from build123d import *

# Parameters (mm, degrees)
BOSS_EXTRUDE1_DEPTH = 90
SKETCH2_R           = 10
CUT_EXTRUDE1_DEPTH  = 90
CUT_EXTRUDE2_DEPTH  = 10
CUT_EXTRUDE3_DEPTH  = 20
SKETCH11_W          = 10
SKETCH11_H          = 9.986072288
BOSS_EXTRUDE2_DEPTH = 70
SKETCH12_W          = 20
SKETCH12_H          = 9.986072288
CUT_EXTRUDE11_DEPTH = 10
CUT_EXTRUDE25_DEPTH = 30
CUT_EXTRUDE26_DEPTH = 30
CUT_EXTRUDE27_DEPTH = 83


with BuildPart() as part:
    # Sketch1 → Boss-Extrude1 (new body)
    with BuildSketch(Plane(origin=(0, 0, 0), x_dir=(1, 0, 0), z_dir=(0, 1, 0))):
        with BuildLine():
            Line((-40, 0), (-30, 0))
            Line((-30, 0), (-30, -30))
            Line((-30, -30), (0, -30))
            Line((0, -30), (20, -50))
            Line((20, -50), (40, -50))
            Line((40, -50), (40, 0))
            ThreePointArc((40, 0), (0, 40), (-40, 0))
        make_face()
    extrude(amount=BOSS_EXTRUDE1_DEPTH)

    # Sketch2 → Cut-Extrude1 (cut)
    with BuildSketch(Plane(origin=(0, 90, 0), x_dir=(1, 0, 0), z_dir=(0, 1, 0))):
        with Locations(Location((0, 0, 0), (0, 0, 270))):
            Circle(SKETCH2_R)
    extrude(amount=-CUT_EXTRUDE1_DEPTH, mode=Mode.SUBTRACT)

    # Sketch3 → Cut-Extrude2 (cut)
    with BuildSketch(Plane(origin=(0, 90, 0), x_dir=(1, 0, 0), z_dir=(0, 1, 0))):
        with BuildLine():
            Line((30, 0), (40, 0))
            Line((40, 0), (40, -40))
            Line((40, -40), (20, -20))
            Line((20, -20), (20, 0))
            ThreePointArc((20, 0), (14.142135624, 14.142135624), (0, 20))
            Line((0, 20), (0, 30))
            ThreePointArc((0, 30), (21.213203436, 21.213203436), (30, 0))
        make_face()
    extrude(amount=-CUT_EXTRUDE2_DEPTH, mode=Mode.SUBTRACT)

    # Sketch4 → Cut-Extrude3 (cut)
    with BuildSketch(Plane(origin=(0, 90, 0), x_dir=(1, 0, 0), z_dir=(0, 1, 0))):
        with BuildLine():
            Line((0, 40), (0, 20))
            ThreePointArc((0, 20), (14.142135624, 14.142135624), (20, 0))
            Line((20, 0), (20, -20))
            Line((20, -20), (20, -59.206848118))
            Line((20, -59.206848118), (-30, -59.206848118))
            Line((-30, -59.206848118), (-30, 0))
            Line((-30, 0), (-40, 0))
            ThreePointArc((-40, 0), (-28.284271247, 28.284271247), (0, 40))
        make_face()
    extrude(amount=-CUT_EXTRUDE3_DEPTH, mode=Mode.SUBTRACT)

    # Sketch11 → Boss-Extrude2 (add)
    with BuildSketch(Plane(origin=(0, 70, 0), x_dir=(1, 0, 0), z_dir=(0, 1, 0))):
        with Locations((-35, -4.993036144)):
            Rectangle(SKETCH11_W, SKETCH11_H)
    extrude(amount=-BOSS_EXTRUDE2_DEPTH)

    # Sketch12 → Cut-Extrude11 (cut)
    with BuildSketch(Plane(origin=(0, 70, 0), x_dir=(1, 0, 0), z_dir=(0, 1, 0))):
        with Locations((-30, -4.993036144)):
            Rectangle(SKETCH12_W, SKETCH12_H)
    extrude(amount=-CUT_EXTRUDE11_DEPTH, mode=Mode.SUBTRACT)

    # Sketch21 → Cut-Extrude25 (cut)
    with BuildSketch(Plane(origin=(0, 70, 0), x_dir=(1, 0, 0), z_dir=(0, 1, 0))):
        with BuildLine():
            Line((-20, 0), (-20, -9.986072288))
            Line((-20, -9.986072288), (-30, -9.986072288))
            Line((-30, -9.986072288), (-30, -30))
            Line((-30, -30), (-20, -30))
            Line((-20, -30), (-20, -44.965046587))
            Line((-20, -44.965046587), (20, -44.965046587))
            Line((20, -44.965046587), (20, 0))
            ThreePointArc((20, 0), (0, 20), (-20, 0))
        make_face()
    extrude(amount=-CUT_EXTRUDE25_DEPTH, mode=Mode.SUBTRACT)

    # Sketch22 → Cut-Extrude26 (cut)
    with BuildSketch(Plane.ZY.offset(30)):
        Polygon((20, 40), (30, 20), (30, 40), align=None)
    extrude(amount=-CUT_EXTRUDE26_DEPTH, mode=Mode.SUBTRACT)

    # 3DSketch3 → Cut-Extrude27 (cut, along a direction that is not the sketch's normal)
    with BuildSketch(Plane(origin=(0, 20, 30), x_dir=(0.549442255794756, 0.8241633836921342, 0.1373605639486891), z_dir=(-0.6666666666666666, 0.3333333333333332, 0.6666666666666669))):
        Polygon((0, 0), (15.109662034, 16.483267674), (28.845718429, -8.241633837), (59.065042498, 24.724901511), (72.801098893, 0), (57.691436858, -16.483267674), (13.736056395, -24.724901511), align=None)
    extrude(amount=CUT_EXTRUDE27_DEPTH, dir=(0, 1, 0), mode=Mode.SUBTRACT)


solid = part.part
Design review of the part built by this model. Coordinates are the model's own, in mm. A direction names the side the tool comes from. Coordinates: 2 decimals unless noted, no trailing zeros. Loops run counter-clockwise (first coordinate to the right, second up) from the corner with the lowest first, then second, coordinate; pieces in that order, holes last. Notation, with made-up numbers: M -25.5,-30.75 L 23.5,-30.75 A25 cw 23.5,-2.75 Z; hole C 30,70.25 d7. An arc over 180 degrees is marked long. Use one line per item in the form item = value.
(1) Draft analysis for pull direction X (two halves, no side actions). For faces 1 (the face through (0, 78, -32)), 2 (the face through (-9.76, 20.28, -2.17)), 3 (the face through (23, 90, -22)), 4 (the face through (-20, 50, 5)), state which applies: pulls with the +X half, pulls with the -X half, needs draft (parallel to the pull), parting line crosses it, or undercut.
Return value:
face_1 = pulls with the -X half
face_2 = undercut
face_3 = needs draft
face_4 = undercut
(2) For faces 5 (the face through (35, 85, 0)), 6 (the face through (-15, 10, 30)), 7 (the face through (-15, 30, 25)), 8 (the face through (20, 60, 15)), list the 3-axis set-ups (+Z, -Z, +X, -X, +Y, -Y) from which the entire face can be reached by the end or side of a thin tool; tool diameter is ignored.
Return value:
face_5 = +Z, +X, -X, +Y
face_6 = +Z, -X, +Y, -Y
face_7 = +Z, -X, +Y
face_8 = +Z, +Y
(3) Consider section D-D (y = 78). Write out the cut boundary in (x, z), and give its area (3 significant figures).
Return value:
outline = M 0,-40 A40 ccw 40,0 L 40,41 L 20,21 L 20,0 A20 cw 0,-20 Z
area = 1,560 mm2
(4) Consider section A-A (y = 9). Write out the cut boundary in (x, z).
Return value:
outline = M -40,0 A40 ccw 40,0 L 40,50 L 20,50 L 0,30 L -30,30 L -30,9.99 L -40,9.99 Z; hole C 0,0 d20
(5) Clearance check with flat-ended pins moving along their axes: P1, Ø12, axis at y = 26, z = 28.5, coming from the -X side; P2, Ø10, axis at y = 32, z = -28.5, coming from the +X side; P3, Ø1, axis at x = -7, y = 30, coming from the -Z side; P4, Ø16, axis at x = 0, z = 0, coming from the -Y side. State where each tip first meets the part, or that it passes through.
Return value:
P1 = -30
P2 = 32.37
P3 = -39.47
P4 = through
(6) Consider section C-C (z = 17). Write out the cut boundary in (x, y), and give its area (3 significant figures).
Return value:
outline = M -30,0 L 40,0 L 40,80 L 20,80 L 20,40 L -30,40 Z
area = 3,600 mm2
(7) For line 1 along X through (y, z) = (45.5, 1); line 2 along X through (y, z) = (23, 0); line 3 along X through (y, z) = (5.5, 23), list the stretches that pass through material, from the lowest coordinate up. Write a range as from..to.
Return value:
line_1 = -40..-20, 20..40
line_2 = -40..-10, 10..40
line_3 = -30..40
(8) Consider section B-B (x = -6.5). Write out the cut boundary in (y, z).
Return value:
outline = M 0,-39.47 L 70,-39.47 L 70,-18.91 L 40,-18.91 L 40,-7.6 L 0,-7.6 Z; M 0,7.6 L 40,7.6 L 40,20 L 20,30 L 0,30 Z
